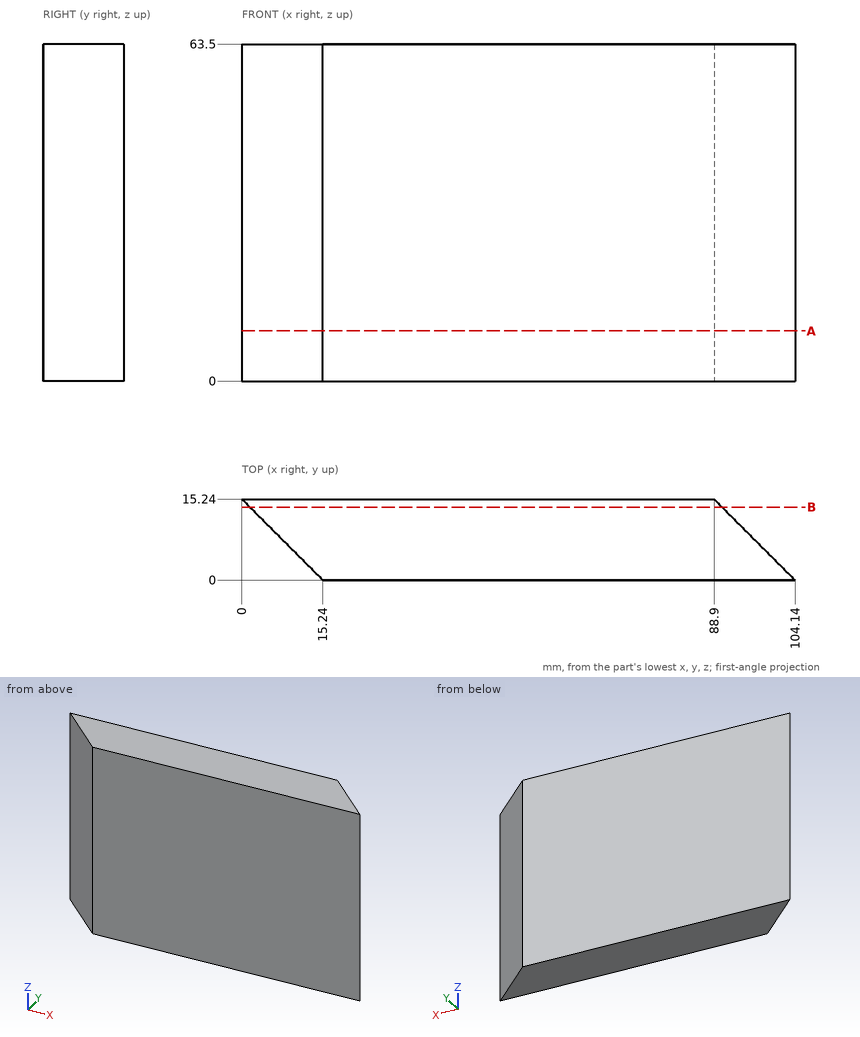
Print and shaded views of the part. All mm, measured from the part's lowest x, y and z. Round coordinates to 2 decimals unless told otherwise and drop trailing zeros. Write each loop counter-clockwise with the first axis right and the second up, starting at its lowest first coordinate (ties: lowest second). Pieces come first, ordered by that corner, then holes.
Item 1: Drop flat-ended pins along their axis: pin 1 Ø1 at (y, z) = (5.5, 49.5) entering from +X; pin 2 Ø2 at (y, z) = (9.5, 47.5) entering from -X; pin 3 Ø3 at (y, z) = (10, 30.5) entering from +X. Give the stop position or say it passes through.
Results:
pin 1: stops at x = 99.14
pin 2: stops at x = 4.74
pin 3: stops at x = 95.64
Item 2: Cut at A-A, the plane z = 9.5. Give the cut face in (x, y).
Results:
outline: (0, 15.24) - (15.24, 0) - (104.14, 0) - (88.9, 15.24) - close
Item 3: Cut at B-B, the plane y = 13.75. Give the cut face in (x, z).
Results:
outline: (1.49, 0) - (90.39, 0) - (90.39, 63.5) - (1.49, 63.5) - close
Item 4: Probe L1, parallel to X at y = 3.5, z = 30.5; L2, parallel to X at y = 14, z = 11; L3, parallel to Y at x = 97, z = 47. List the from-to ranges inside material, lowest first.
Results:
L1: x = 11.74 to 100.64
L2: x = 1.24 to 90.14
L3: y = 0 to 7.14
